Source: CAD feature listing. Evaluate the final solid. Frame: model axes, mm. A direction names the side the tool comes from. Round coordinates to 2 decimals unless told otherwise and drop trailing zeros. Order: outer loops, then holes, each group sorted by start corner. A loop starts at its lowest first (then second) coordinate and runs counter-clockwise, first axis right, second up. Notation, with made-up numbers: (-12, -23.75) - (-6, -23.75) arc R23 cw to (-6, 10.25) - close; hole circle Ø2 at (9, 1). An arc over 180 degrees is marked (long way). Return JSON: item names as keys, results as strings. Group by question number.
1) Section B-B, the plane x = 1.75. Return loops of the section in (y, z), plus the area to 3 significant figures.
2) Section C-C, the plane y = 13.5. Return loops of the section in (x, z).
3) Section A-A, the plane z = -6.5. Return loops of the section in (x, y), plus the area to 4 significant figures.
4) Section D-D, the plane x = 0. Return loops of the section in (y, z) (3 decimals).
5) Ray query, line 1 (Z direction, x = 0.1, y = 15.6) (3 decimals); line 2 (Z direction, x = 0.4, y = -16.1); line 3 (Y direction, x = 1.5, z = -8.5). Return the intervals inside material, ascending. Write a range as from..to.
6) Access query for faces 4 (the flat face through (0.5, 3.3, -11.43)), 5 (the flat face through (4, 7, -3.43)), 6 (the flat face through (2, 15, 4)). Directions: +Z, -Z, +X, -X, +Y, -Y. A direction counts if a zero-diameter tool reaches every point of the face in a straight line with its end or side. Return the directions, or none.
7) Mould query, pull axis Z, two halves, no side actions, for faces 1 (the cylindrical face through (0.01, 14.35, -8.77)), 2 (the flat face through (2, 15, -4)), 3 (the flat face through (1, 18.1, 0)). Classes: pulls with the +Z half, pulls with the -Z half, needs draft (parallel to the pull), parting line crosses it, or undercut.
8) Contact query for flat-ended pins moving along their axis: P1, Ø0.8, axis at x = 2.5, z = -1, coming from the -Y side; P2, Ø12, axis at y = -13, z = 3.5, coming from the +X side; P3, Ø1.2, axis at x = 2.5, y = 15, coming from the -Z side; P4, Ø2, axis at y = 15.6, z = -8.825, coming from the +X side. Output: stop coordinate, or through.
```python
from build123d import *

# Parameters (mm, degrees)
F0_W     = 36.2
F0_H     = 22.86
F1_DEPTH = 0.75
F2_W     = 8
F2_H     = 8
F3_DEPTH = 5.75
F2_W_2   = 5.75
F4_DEPTH = 2.5
F5_R     = 2.25
F6_R     = 1.25
F7_DEPTH = 1.5


with BuildPart() as f1:
    # F0 (on Right) → F1 (new body, symmetric)
    with BuildSketch(Plane.YZ):
        Rectangle(F0_W, F0_H)
    extrude(amount=F1_DEPTH, both=True)

    # F2 (on face) → F3 (join)
    with BuildSketch(Plane.YZ.offset(0.75)):
        with Locations((7.3, -7.43)):
            Rectangle(F2_W, F2_H)
    extrude(amount=F3_DEPTH)

    # F2 (on face) → F4 (join)
    with BuildSketch(Plane.YZ.offset(0.75)):
        with Locations((15.225, 0)):
            Rectangle(F2_W_2, F2_H)
    extrude(amount=F4_DEPTH)

    # F5
    f5_edges = [f1.edges().sort_by_distance(p)[0] for p in [
        (0, -18.1, 11.43),
        (0, 18.1, 11.43),
        (0, 18.1, -11.43),
        (0, -18.1, -11.43),
    ]]
    fillet(f5_edges, radius=F5_R)

    # F6 (on face) → F7 (cut, through all)
    with BuildSketch(Plane.YZ.offset(0.75)):
        with Locations((15.6, 8.825)):
            Circle(F6_R)
        with Locations((15.6, -8.825)):
            Circle(F6_R)
        with Locations((-16.1, 6.5)):
            Circle(F6_R)
        with Locations((-16.1, -6.5)):
            Circle(F6_R)
    extrude(amount=-F7_DEPTH, mode=Mode.SUBTRACT)


solid = f1.part
```
Geometry check:
{
 "1": {"outline": "(3.3, -11.43) - (11.3, -11.43) - (11.3, -3.43) - (3.3, -3.43) - close; (12.35, -4) - (18.1, -4) - (18.1, 4) - (12.35, 4) - close", "area": "110 mm2"},
 "2": {"outline": "(-0.75, -11.43) - (0.75, -11.43) - (0.75, -4) - (3.25, -4) - (3.25, 4) - (0.75, 4) - (0.75, 11.43) - (-0.75, 11.43) - close"},
 "3": {"outline": "(-0.75, -18.1) - (0.75, -18.1) - (0.75, -17.35) - (-0.75, -17.35) - close; (-0.75, -14.85) - (0.75, -14.85) - (0.75, 3.3) - (6.5, 3.3) - (6.5, 11.3) - (0.75, 11.3) - (0.75, 18.1) - (-0.75, 18.1) - close", "area": "96.55 mm2"},
 "4": {"outline": "(-18.1, -9.18) arc R2.25 ccw to (-15.85, -11.43) - (15.85, -11.43) arc R2.25 ccw to (18.1, -9.18) - (18.1, 9.18) arc R2.25 ccw to (15.85, 11.43) - (-15.85, 11.43) arc R2.25 ccw to (-18.1, 9.18) - close; hole circle Ø2.5 at (-16.1, -6.5); hole circle Ø2.5 at (-16.1, 6.5); hole circle Ø2.5 at (15.6, -8.825); hole circle Ø2.5 at (15.6, 8.825)"},
 "5": {"line 1": "-11.43..-10.075, -7.575..7.575, 10.075..11.43", "line 2": "-11.42..-7.75, -5.25..5.25, 7.75..11.42", "line 3": "3.3..11.3"},
 "6": {"face 4": "-Z, +X, -X, +Y, -Y", "face 5": "+Z, +X, -Y", "face 6": "+Z, +X, +Y, -Y"},
 "7": {"face 1": "undercut", "face 2": "pulls with the -Z half", "face 3": "needs draft"},
 "8": {"P1": "y = 12.35", "P2": "x = 0.75", "P3": "z = -4", "P4": "through"}
}
